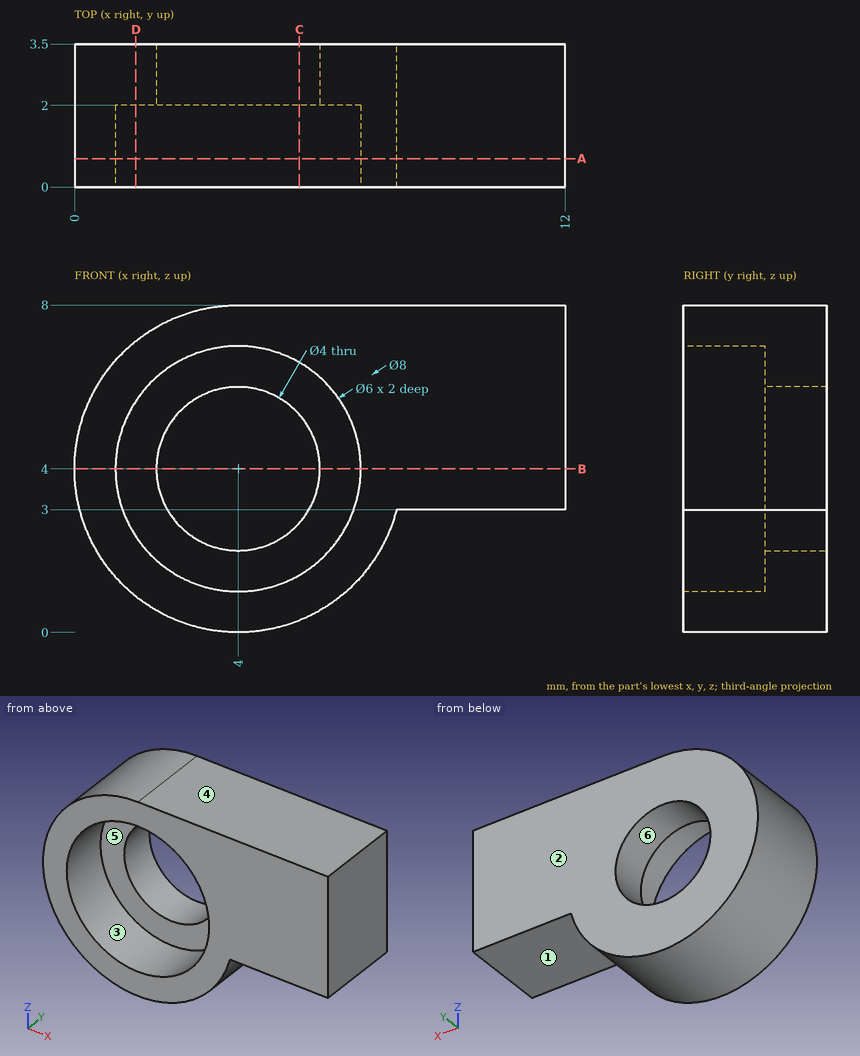
Can you work these out from the drawing? Everything is in mm from the part's minimum corner. A direction names the side the tool comes from. Round coordinates to 2 decimals unless told otherwise and drop trailing zeros. Loops run counter-clockwise (first coordinate to the right, second up) from the corner with the lowest first, then second, coordinate; pieces in that order, holes last. Notation, with made-up numbers: (3, 85) - (31, 85) arc R26 cw to (31, 115) - close; hole circle Ø4 at (14, -39.5). An arc over 180 degrees is marked (long way). Write item = value, one per line. Start each with the question number.
(1) If we section it at B-B (z = 4): Please give me the cut outline in (x, y).
(2) If we mould it in two halves opening along Z, with no side actions, what happens to the marked faces 1, 2, 3 and 4? For each: released by +Z, released by -Z, zero draft, split by the parting line, or undercut.
(3) For P1, Ø1, axis at y = 2, z = 7, coming from the -X side, with a flat end and sliding along its axis, tell me the tip position at first contact or that it passes through.
(4) If we section it at D-D (x = 1.5): Please give me the cut outline in (y, z), and give its area (3 significant figures).
(5) If we section it at A-A (y = 0.7): Please give me the cut outline in (x, z), and give its area (3 significant figures).
(6) If we section it at C-C (x = 5.5): Please give me the cut outline in (y, z).
(7) If I drill on probe 1 along X at (y, z) = (0.95, 4); probe 2 along X at (y, z) = (2.35, 4); probe 3 along Z at (x, y) = (8, 0.9), over which ranges is the centre line in solid material (lowest first)? Write a range as [from, to].
(8) For the marked faces 5 and 6, which set-ups out of +Z, -Z, +X, -X, +Y, -Y let a thin tool reach every point of the face, with its end or its side?
Ans:
q1.outline = (0, 0) - (1, 0) - (1, 2) - (2, 2) - (2, 3.5) - (0, 3.5) - close; (6, 2) - (7, 2) - (7, 0) - (12, 0) - (12, 3.5) - (6, 3.5) - close
q2.face_1 = released by -Z
q2.face_2 = zero draft
q2.face_3 = undercut
q2.face_4 = released by +Z
q3.P1 = 0.88
q4.outline = (0, 0.88) - (3.5, 0.88) - (3.5, 7.12) - (0, 7.12) - (0, 5.66) - (2, 5.66) - (2, 2.34) - (0, 2.34) - close
q4.area = 15.2 mm²
q5.outline = (4, 8) arc R4 ccw (long way) to (7.87, 3) - (12, 3) - (12, 8) - close; hole circle Ø6 at (4, 4)
q5.area = 45.5 mm²
q6.outline = (0, 0.29) - (3.5, 0.29) - (3.5, 2.68) - (2, 2.68) - (2, 1.4) - (0, 1.4) - close; (0, 6.6) - (2, 6.6) - (2, 5.32) - (3.5, 5.32) - (3.5, 8) - (0, 8) - close
q7.probe_1 = [0, 1], [7, 12]
q7.probe_2 = [0, 2], [6, 12]
q7.probe_3 = [3, 8]
q8.face_5 = -Y
q8.face_6 = +Y, -Y
